from build123d import *

# Parameters (mm, degrees)
PAD087_DEPTH          = 4.5
POLARPATTERN008_COUNT = 4
PAD088_DEPTH          = 2
POLARPATTERN009_COUNT = 4


with BuildPart() as part:
    # Sketch179 → Pad087 (new body)
    with BuildSketch(Plane.XY):
        with BuildLine():
            Line((0, 0), (0, 10))
            Line((-8.75, 10), (0, 10))
            ThreePointArc((-8.75, 10), (-9.633883, 9.633883), (-10, 8.75))
            Line((-10, 0), (-10, 8.75))
            Line((0, 0), (-10, 0))
        make_face()
    pad087 = extrude(amount=PAD087_DEPTH)

    # PolarPattern008: Pad087 ×4 about axis
    polarpattern008_axis = Axis((0, 0, 0), (0, 0, 1))
    for i in range(1, POLARPATTERN008_COUNT):
        add(pad087.rotate(polarpattern008_axis, i * 360 / POLARPATTERN008_COUNT))

    # Sketch178 → Pad088 (join)
    with BuildSketch(Plane.XY):
        Polygon((-5.7, 7.124264), (-2.875736, 4.3), (2.875736, 4.3), (5.7, 7.124264), (5.7, 7.7), (-5.7, 7.7), align=None)
    pad088 = extrude(amount=-PAD088_DEPTH)

    # PolarPattern009: Pad088 ×4 about axis
    polarpattern009_axis = Axis((0, 0, 0), (0, 0, 1))
    for i in range(1, POLARPATTERN009_COUNT):
        add(pad088.rotate(polarpattern009_axis, i * 360 / POLARPATTERN009_COUNT))


solid = part.part
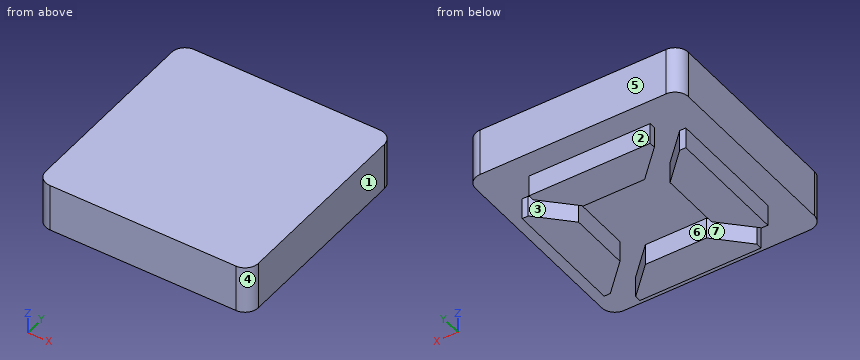
Input: part model. Units: mm. Frame: model coordinates. Face numbers are marked on the shaded views. A direction names the side the tool comes from. Coordinates: 2 decimals unless noted, no trailing zeros. Loops run counter-clockwise (first coordinate to the right, second up) from the corner with the lowest first, then second, coordinate; pieces in that order, holes last. Notation, with made-up numbers: (-26, 76.25) -> (11, 76.25) arc R14 ccw to (11, 92.25) -> close; hole circle Ø1 at (-15.75, -29.75). An arc over 180 degrees is marked (long way). Write item = value, one per line. Start each with the question number.
Item 1: Material intervals for line 1 (Y direction, x = -1.5, z = -0.75); line 2 (X direction, y = -5, z = -1.5), sorted ascending.
Item 2: Cut plane A-A, the plane z = -1.25. Return loops of the section in (x, y).
Item 3: Mould query, pull axis X, two halves, no side actions, for the marked faces 4, 5, 6 and 7. Classes: pulls with the +X half, pulls with the -X half, needs draft (parallel to the pull), parting line crosses it, or undercut.
Item 4: First-contact query: P1, Ø0.5, axis at y = 7.5, z = -1.5, coming from the -X side; P2, Ø0.6, axis at x = -7.5, z = -1, coming from the +Y side; P3, Ø0.6, axis at y = -2.5, z = -1, coming from the -X side. Flat tips, straight axial feed; report the tip coordinate or a pass-through.
Item 5: Cut plane D-D, the plane y = 6.5. Return loops of the section in (x, z), plus the area to 3 significant figures.
Item 6: Cut plane B-B, the plane x = -0.75. Return loops of the section in (y, z), plus the area to 3 significant figures.
Item 7: Reachability of the marked faces 1, 2 and 3 from +Z, -Z, +X, -X, +Y, -Y: full face, straight path, thin tool, end or side. Return the list, or none.
Ans:
q1.line_1 = -7.7 to -4.3, 4.3 to 7.7
q1.line_2 = -7.7 to -6.42, -3.58 to 3.58, 6.42 to 7.7
q2.outline = (-7.7, -5.7) -> (-7.12, -5.7) -> (-4.3, -2.88) -> (-4.3, 2.88) -> (-7.12, 5.7) -> (-7.7, 5.7) -> close; (-5.7, -7.7) -> (5.7, -7.7) -> (5.7, -7.12) -> (2.88, -4.3) -> (-2.88, -4.3) -> (-5.7, -7.12) -> close; (-5.7, 7.12) -> (-2.88, 4.3) -> (2.88, 4.3) -> (5.7, 7.12) -> (5.7, 7.7) -> (-5.7, 7.7) -> close; (4.3, -2.88) -> (7.12, -5.7) -> (7.7, -5.7) -> (7.7, 5.7) -> (7.12, 5.7) -> (4.3, 2.88) -> close
q3.face_4 = pulls with the +X half
q3.face_5 = needs draft
q3.face_6 = undercut
q3.face_7 = undercut
q4.P1 = -5.7
q4.P2 = 5.7
q4.P3 = -7.7
q5.outline = (-10, 0) -> (-5.08, 0) -> (-5.08, -2) -> (5.08, -2) -> (5.08, 0) -> (10, 0) -> (10, 4.5) -> (-10, 4.5) -> close
q5.area = 110 mm²
q6.outline = (-10, 0) -> (-7.7, 0) -> (-7.7, -2) -> (-4.3, -2) -> (-4.3, 0) -> (4.3, 0) -> (4.3, -2) -> (7.7, -2) -> (7.7, 0) -> (10, 0) -> (10, 4.5) -> (-10, 4.5) -> close
q6.area = 104 mm²
q7.face_1 = +Z, -Z, +X, +Y, -Y
q7.face_2 = -Z, +X, -X, +Y
q7.face_3 = -Z
